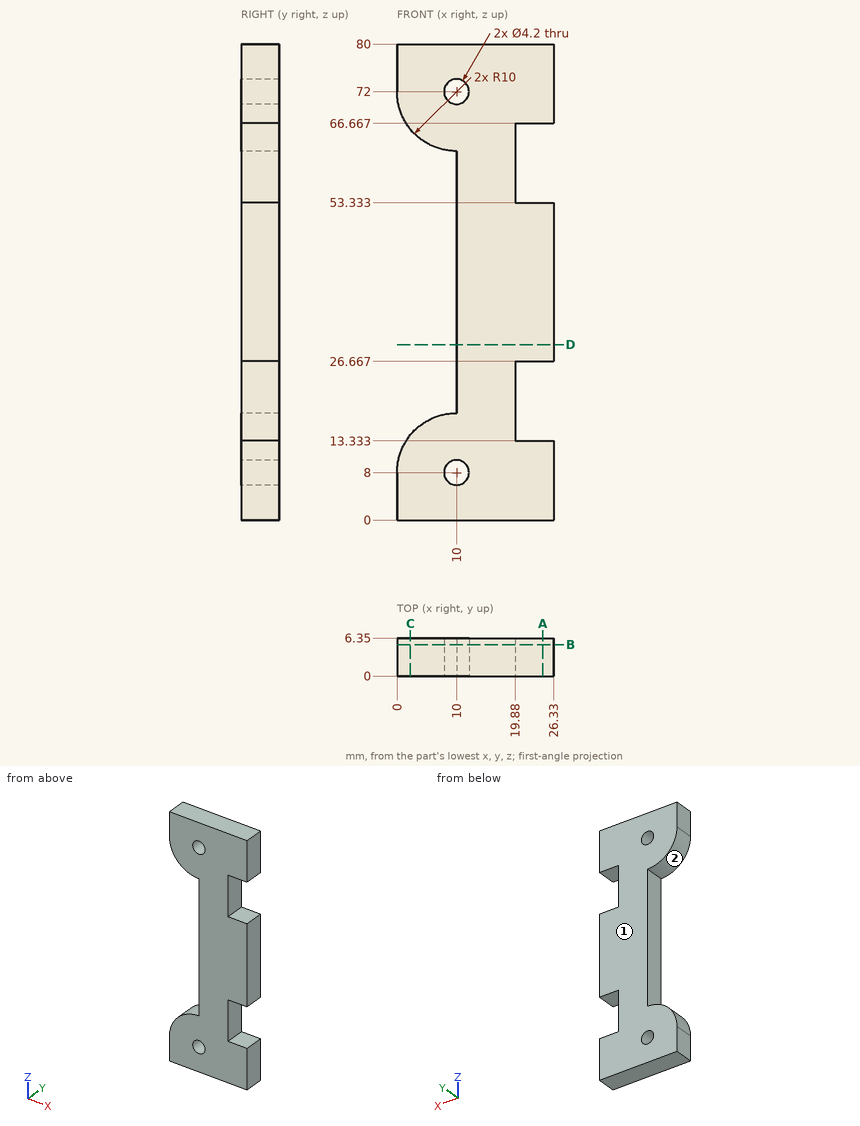
For this review, use the dimensioned drawing (mm, ordinates from the lowest corner) and the shaded views. Round coordinates to 2 decimals unless told otherwise and drop trailing zeros. Order: outer loops, then holes, each group sorted by start corner. A loop starts at its lowest first (then second) coordinate and runs counter-clockwise, first axis right, second up.
1) Clearance check with flat-ended pins moving along their axes: pin 1 Ø6 at (x, z) = (12.5, 62) entering from -Y; pin 2 Ø3.5 at (x, z) = (10, 8) entering from +Y; pin 3 Ø3 at (y, z) = (2.5, 50) entering from -X; pin 4 Ø3 at (y, z) = (1, 65) entering from +X. State where each tip first meets the part, or that it passes through.
The answers:
pin 1: stops at y = 0
pin 2: passes through
pin 3: stops at x = 10
pin 4: stops at x = 19.88
2) Consider section D-D (z = 29.5). State the section outline as (x, y) points, plus the area to 3 significant figures.
The answers:
outline: (10, 0) - (26.33, 0) - (26.33, 6.35) - (10, 6.35) - close
area: 104 mm2
3) Consider section B-B (y = 5.25). State the section outline as (x, z) points, plus the area to 3 significant figures.
The answers:
outline: (0, 0) - (26.33, 0) - (26.33, 13.33) - (19.88, 13.33) - (19.88, 26.67) - (26.33, 26.67) - (26.33, 53.33) - (19.88, 53.33) - (19.88, 66.67) - (26.33, 66.67) - (26.33, 80) - (0, 80) - (0, 72) arc R10 ccw to (10, 62) - (10, 18) arc R10 ccw to (0, 8) - close; hole circle Ø4.2 at (10, 8); hole circle Ø4.2 at (10, 72)
area: 1,420 mm2
4) Draft analysis for pull direction Z (two halves, no side actions). For the marked faces 1 and 2, state which applies: released by +Z, released by -Z, zero draft, split by the parting line, or undercut.
The answers:
face 1: zero draft
face 2: undercut
5) Consider section C-C (x = 2.25). State the section outline as (y, z) points.
The answers:
outline: (0, 0) - (6.35, 0) - (6.35, 14.32) - (0, 14.32) - close; (0, 65.68) - (6.35, 65.68) - (6.35, 80) - (0, 80) - close
6) Consider section A-A (x = 24.5). State the section outline as (y, z) points.
The answers:
outline: (0, 0) - (6.35, 0) - (6.35, 13.33) - (0, 13.33) - close; (0, 26.67) - (6.35, 26.67) - (6.35, 53.33) - (0, 53.33) - close; (0, 66.67) - (6.35, 66.67) - (6.35, 80) - (0, 80) - close
7) For L1, parallel to X at y = 3.5, z = 8; L2, parallel to X at y = 2.5, z = 45; L3, parallel to X at y = 4, z = 24.5, list the stretches that pass through material, from the lowest coordinate up.
The answers:
L1: x = 0 to 7.9, 12.1 to 26.33
L2: x = 10 to 26.33
L3: x = 10 to 19.88
